Geometry check sheet. Reference: the model listing, model coordinates, mm. A direction names the side the tool comes from. Give positions to 0.01 mm unless a question says otherwise; leave off trailing zeros. Loops run counter-clockwise (first coordinate to the right, second up) from the corner with the lowest first, then second, coordinate; pieces in that order, holes last.
1. Material ranges on L1, parallel to Y at x = 50, z = -62.5; L2, parallel to Y at x = -19.5, z = 75; L3, parallel to X at y = 37, z = -47, recorded low to high.
2. Cross-section at B-B, the plane y = -91. Record the cut outline in (x, z).
3. Go/stop test with flat-tipped pins: pin 1 Ø23 at (y, z) = (-38, 24.5) entering from -X; pin 2 Ø1.5 at (x, z) = (-29.5, -46) entering from -Y; pin 3 Ø7 at (y, z) = (-83, 29.5) entering from +X. Record where each tip stops, or that it passes through.
4. Cross-section at D-D, the plane y = 3. Record the cut outline in (x, z), plus the area to 3 significant figures.
5. Cross-section at C-C, the plane z = -17. Record the cut outline in (x, y).
6. Cross-section at A-A, the plane x = 39. Record the cut outline in (y, z).
7. Tool access check on faces 1 (the flat face through (-62, 0, -27)), 2 (the flat face through (-15.965, -89, 3)), 3 (the flat face through (100, 23, 0)), 4 (the flat face through (-9.41, -88.722, 45.105)), 5 (the flat face through (66, -4, 0)). Record the directions out of +Z, -Z, +X, -X, +Y, -Y that give a thin tool (end or side, any length) a straight path to the whole face; none if there is none.
from build123d import *

# Parameters (mm, degrees)
F0_W     = 127
F0_H     = 127
F1_DEPTH = 76.2
F2_W     = 229.4309809804
F2_H     = 45.7849353552
F3_DEPTH = 127
F4_W     = 129.2693130672
F4_H     = 54.8701006919
F5_DEPTH = 76.2
F6_W     = 24.2228312418
F6_H     = 11.9455056265
F7_DEPTH = 101.6


with BuildPart() as f1:
    # F0 (on Front) → F1 (new body)
    with BuildSketch(Plane.XZ):
        with Locations((-2.1202601492, 8.4589998459)):
            Rectangle(F0_W, F0_H)
    extrude(amount=F1_DEPTH)

    # F2 (on Top) → F3 (join)
    with BuildSketch(Plane.XY):
        with Locations((16.3871459663, 22.8924676776)):
            Rectangle(F2_W, F2_H)
    extrude(amount=F3_DEPTH)

    # F4 (on Top) → F5 (join)
    with BuildSketch(Plane.XY):
        with Locations((5.9114117175, 18.4862976894)):
            Rectangle(F4_W, F4_H)
    extrude(amount=-F5_DEPTH)

    # F6 (on Front) → F7 (join)
    with BuildSketch(Plane.XZ):
        Polygon((8.2575650886, 53.4568582272), (-27.5789517909, 36.5159586072), (-15.9652661532, 36.5159586072), (8.2575650886, 47.7774481696), align=None)
        Polygon((-15.9652661532, 36.5159586072), (-27.5789517909, 36.5159586072), (-27.5789517909, -3.3023932483), (-15.9652661532, -3.3023932483), (-15.9652661532, 10.3022092953), (-15.9652661532, 22.2477149218), align=None)
        Polygon((8.2575650886, 54.1023947299), (8.2575650886, 53.4568582272), (8.2575650886, 47.7774481696), (21.8621697277, 54.1023947299), align=None)
        with Locations((-3.8538505323, 16.2749621086)):
            Rectangle(F6_W, F6_H)
        Polygon((21.8621697277, 54.1023947299), (8.2575650886, 47.7774481696), (8.2575650886, 22.2477149218), (8.2575650886, 10.3022092953), (21.8621697277, 10.3022092953), align=None)
    extrude(amount=F7_DEPTH)


solid = f1.part
Result:
1. L1: y = -8.95 to 45.92
1. L2: y = 0 to 45.78
1. L3: x = -58.72 to 70.55
2. outline: (-27.58, -3.3) - (-15.97, -3.3) - (-15.97, 10.3) - (21.86, 10.3) - (21.86, 54.1) - (8.26, 54.1) - (8.26, 53.46) - (-27.58, 36.52) - close; hole (-15.97, 22.25) - (8.26, 22.25) - (8.26, 47.78) - (-15.97, 36.52) - close
3. pin 1: stops at x = -65.62
3. pin 2: stops at y = -76.2
3. pin 3: stops at x = 21.86
4. outline: (-98.33, 0) - (-58.72, 0) - (-58.72, -76.2) - (70.55, -76.2) - (70.55, 0) - (131.1, 0) - (131.1, 127) - (-98.33, 127) - close
4. area: 39,000 mm2
5. outline: (-65.62, -76.2) - (61.38, -76.2) - (61.38, -8.95) - (70.55, -8.95) - (70.55, 45.92) - (-58.72, 45.92) - (-58.72, 0) - (-65.62, 0) - close
6. outline: (-76.2, -55.04) - (-8.95, -55.04) - (-8.95, -76.2) - (45.92, -76.2) - (45.92, 0) - (45.78, 0) - (45.78, 127) - (0, 127) - (0, 71.96) - (-76.2, 71.96) - close
7. face 1: -Z, -X, +Y
7. face 2: -Z, +X, -Y
7. face 3: -Z, +X, +Y, -Y
7. face 4: +Z, -X, -Y
7. face 5: +Z, +X, -Y
